```python
from build123d import *

# Parameters (mm, degrees)
SKETCH_1_W          = 48
SKETCH_1_H          = 20
EXTRUDE_1_DEPTH     = 30
SKETCH_2_W          = 14
SKETCH_2_H          = 30
CUT_EXTRUDE_1_DEPTH = 7
SKETCH_7_W          = 22
SKETCH_7_H          = 30
EXTRUDE_2_DEPTH     = 48
SKETCH_8_W          = 21
SKETCH_8_H          = 30
CUT_EXTRUDE_2_DEPTH = 14
SKETCH_9_W          = 21
SKETCH_9_H          = 30
CUT_EXTRUDE_3_DEPTH = 14
SKETCH_11_W         = 10.2
SKETCH_11_H         = 20.2
CUT_EXTRUDE_4_DEPTH = 56.497747702
SKETCH_13_R         = 4.1
CUT_EXTRUDE_5_DEPTH = 44.783558558
FILLET_1_R          = 7
SKETCH1_W           = 10.2
SKETCH1_H           = 20.2
BOSS_EXTRUDE1_DEPTH = 4
SKETCH2_W           = 20
SKETCH2_H           = 21
CUT_EXTRUDE1_DEPTH  = 51


with BuildPart() as part:
    # Эскиз1 → Бобышка-Вытянуть1 (new body)
    with BuildSketch(Plane(origin=(0, 0, 0), x_dir=(1, 0, 0), z_dir=(0, 1, 0))):
        Rectangle(SKETCH_1_W, SKETCH_1_H)
    extrude(amount=EXTRUDE_1_DEPTH)

    # Эскиз2 → Вырез-Вытянуть1 (cut)
    with BuildSketch(Plane.XY.offset(10)):
        with Locations((0, 15)):
            Rectangle(SKETCH_2_W, SKETCH_2_H)
    extrude(amount=-CUT_EXTRUDE_1_DEPTH, mode=Mode.SUBTRACT)

    # Эскиз7 → Бобышка-Вытянуть2 (add)
    with BuildSketch(Plane(origin=(24, 0, 0), x_dir=(0, 0, -1), z_dir=(1, 0, 0))):
        with Locations((21, 15)):
            Rectangle(SKETCH_7_W, SKETCH_7_H)
    extrude(amount=-EXTRUDE_2_DEPTH)

    # Эскиз8 → Вырез-Вытянуть2 (cut)
    with BuildSketch(Plane(origin=(24, 0, 0), x_dir=(0, 0, -1), z_dir=(1, 0, 0))):
        with Locations((21.5, 15)):
            Rectangle(SKETCH_8_W, SKETCH_8_H)
    extrude(amount=-CUT_EXTRUDE_2_DEPTH, mode=Mode.SUBTRACT)

    # Эскиз9 → Вырез-Вытянуть3 (cut)
    with BuildSketch(Plane.ZY.offset(24)):
        with Locations((-21.5, 15)):
            Rectangle(SKETCH_9_W, SKETCH_9_H)
    extrude(amount=-CUT_EXTRUDE_3_DEPTH, mode=Mode.SUBTRACT)

    # Эскиз11 → Вырез-Вытянуть4 (cut, through all)
    with BuildSketch(Plane.ZY.offset(10)):
        with Locations((-21.5, 15)):
            Rectangle(SKETCH_11_W, SKETCH_11_H)
    extrude(amount=-CUT_EXTRUDE_4_DEPTH, mode=Mode.SUBTRACT)

    # Эскиз13 → Вырез-Вытянуть5 (cut, through all)
    with BuildSketch(Plane(origin=(0, 0, -11), x_dir=(-1, 0, 0), z_dir=(0, 0, -1))):
        with Locations((17, 15)):
            Circle(SKETCH_13_R)
        with Locations((-17, 15)):
            Circle(SKETCH_13_R)
    extrude(amount=-CUT_EXTRUDE_5_DEPTH, mode=Mode.SUBTRACT)

    # Скругление1
    fillet_1_edges = [part.edges().sort_by_distance(p)[0] for p in [
        (-7, 15, 3),
        (7, 15, 3),
    ]]
    fillet(fillet_1_edges, radius=FILLET_1_R - 0.0001)  # a hair under: the kernel refuses the full size

    # Sketch1 → Boss-Extrude1 (add)
    with BuildSketch(Plane(origin=(10, 0, 0), x_dir=(0, 0, -1), z_dir=(1, 0, 0))):
        with Locations((21.5, 15)):
            Rectangle(SKETCH1_W, SKETCH1_H)
    extrude(amount=-BOSS_EXTRUDE1_DEPTH)

    # Sketch2 → Cut-Extrude1 (cut, through all)
    with BuildSketch(Plane(origin=(0, 30, 0), x_dir=(1, 0, 0), z_dir=(0, 1, 0))):
        with Locations((0, 21.5)):
            Rectangle(SKETCH2_W, SKETCH2_H)
    extrude(amount=-CUT_EXTRUDE1_DEPTH, mode=Mode.SUBTRACT)


solid = part.part
```
Here's how the part is built. I have some questions about the finished solid (model axes, mm). A direction names the side the tool comes from. Coordinates: 2 decimals unless noted, no trailing zeros. Order: outer loops, then holes, each group sorted by start corner. A loop starts at its lowest first (then second) coordinate and runs counter-clockwise, first axis right, second up.
Item 1: If we section it at C-C, the plane z = 6: List the corners of the cut face in (x, y) for me.
Response values:
outline: (-24, 0) - (-5.74, 0) - (-5.74, 30) - (-24, 30) - close; (5.74, 0) - (24, 0) - (24, 30) - (5.74, 30) - close; hole circle Ø8.2 at (-17, 15); hole circle Ø8.2 at (17, 15)
Item 2: If we section it at B-B, the plane y = 15: Give the number of separate pieces and of enclosed holes in the cut face, then the cut area to 3 significant figures.
Response values:
separate pieces: 3
enclosed holes: 0
area: 587 mm2
Item 3: If we section it at A-A, the plane x = 17: List the corners of the cut face in (y, z) for me, then the cut area to 3 significant figures.
Response values:
outline: (0, -11) - (10.9, -11) - (10.9, 10) - (0, 10) - close; (19.1, -11) - (30, -11) - (30, 10) - (19.1, 10) - close
area: 458 mm2
Item 4: I need wall thicknesses on probe 1 along Y at (x, z) = (17, 2.75); probe 2 along X at (y, z) = (15.5, 5.5); probe 3 along X at (y, z) = (18.25, 2.75). Which ranges of each line are inside material? Lowest first, please.
Response values:
probe 1: y = 0 to 10.9, 19.1 to 30
probe 2: x = -24 to -21.07, -12.93 to -5.36, 5.36 to 12.93, 21.07 to 24
probe 3: x = -24 to -19.5, -14.5 to 14.5, 19.5 to 24
Item 5: Which directions (+Z, -Z, +X, -X, +Y, -Y) give clear straight access to the entire face, cutting with the end or side of a thin tool? Please do faces 4 (the face through (0, 30, 0)), 5 (the face through (4.9, 15.2, 5)).
Response values:
face 4: +Z, -Z, +X, -X, +Y
face 5: +Z, +Y, -Y
Item 6: Thinking about a two-plate mould opening in X: for faces 1 (the face through (-12, 15, 10)), 2 (the face through (24, 15, 0)), 3 (the face through (21.096, 15.18, -0.647)), which applies, pulls with the +X half, pulls with the -X half, needs draft (parallel to the pull), parting line crosses it, or undercut?
Response values:
face 1: needs draft
face 2: pulls with the +X half
face 3: undercut
